CAD build for the part. Positions are in the model's coordinates, mm. Coordinates: 2 decimals unless noted, no trailing zeros. Order: outer loops, then holes, each group sorted by start corner. A loop starts at its lowest first (then second) coordinate and runs counter-clockwise, first axis right, second up. Notation, with made-up numbers: (76, -36) - (108, -36) arc R16 ccw to (108, -17) - close; hole circle Ø9 at (81.5, 85.5). An arc over 180 degrees is marked (long way). Return JSON: item names as keys, results as strings.
Autodesk Inventor part; units mm, degrees
ref_plane "YZ Plane" through (0, 0, 0) normal (1, 0, 0) x (0, 1, 0)
ref_plane "XZ Plane" through (0, 0, 0) normal (0, 1, 0) x (-1, 0, 0)
ref_plane "XY Plane" through (0, 0, 0) normal (0, 0, 1) x (1, 0, 0)
sketch "Sketch1" plane through (0, 0, 0) normal (0, 1, 0) x (-1, 0, 0)
  line L0 (6.35, -3.6662) -> (0, -7.3323)
  line L1 (0, -7.3323) -> (-6.35, -3.6662)
  line L2 (-6.35, -3.6662) -> (-6.35, 3.6662)
  line L3 (-6.35, 3.6662) -> (0, 7.3323)
  line L4 (0, 7.3323) -> (6.35, 3.6662)
  line L5 (6.35, 3.6662) -> (6.35, -3.6662)
  point P0 (0, 0)
  point P1 (0, 0)
  point P2 (0, 0)
  dimension "d0" = 12.7
extrude "Extrusion1" add sketch "Sketch1" along normal blind 673.1
hole "Hole1" at (0, 0, 0) direction (0, 1, 0) diameter 4.9784 depth 25.4
sketch "Sketch2" plane through (0, 673.1, 0) normal (0, 1, 0) x (1, 0, 0)
  point P0 (0, 0)
  point P1 (0, 0)
hole "Hole2" at (0, 673.1, 0) direction (0, -1, 0) diameter 4.9784 depth 25.4
properties part number "Intake Roller Hex Shaft"
Item 1: Mould opens along Y. For faces 1 (the flat face through (0, 673.1, -3)), 2 (the flat face through (0, 0, -3)) say: released by +Y, released by -Y, zero draft, split by the parting line, or undercut.
Findings below:
{"face 1": "released by +Y", "face 2": "released by -Y"}
Item 2: Wall check: L1, parallel to X at y = 16, z = 0; L2, parallel to Z at x = 0, y = 666.5; L3, parallel to Z at x = 1.75, y = 75. Give the ranges that are in metal, low to high. Write a range as [from, to].
Findings below:
{"L1": "x = [-6.35, -2.49], [2.49, 6.35]", "L2": "z = [-7.33, -2.49], [2.49, 7.33]", "L3": "z = [-6.32, 6.32]"}
Item 3: Band-saw the part on B-B, the plane y = 81.5. List the corners of the cut face in (x, z), then the cut area to 3 significant figures.
Findings below:
{"outline": "(-6.35, -3.67) - (0, -7.33) - (6.35, -3.67) - (6.35, 3.67) - (0, 7.33) - (-6.35, 3.67) - close", "area": "140 mm²"}
Item 4: Band-saw the part on A-A, the plane z = 0. List the corners of the cut face in (x, y), then the cut area to 3 significant figures.
Findings below:
{"outline": "(-6.35, 0) - (-2.49, 0) - (-2.49, 25.4) - (2.49, 25.4) - (2.49, 0) - (6.35, 0) - (6.35, 673.1) - (2.49, 673.1) - (2.49, 647.7) - (-2.49, 647.7) - (-2.49, 673.1) - (-6.35, 673.1) - close", "area": "8,300 mm²"}
Item 5: Drop flat-ended pins along their axis: P1, Ø2.5, axis at x = 0, z = -0.5, coming from the -Y side; P2, Ø4, axis at x = 1, y = 445.5, coming from the -Z side; P3, Ø2.5, axis at x = 0, z = -0.5, coming from the +Y side. Give the stop position or say it passes through.
Findings below:
{"P1": "stops at y = 25.4", "P2": "stops at z = -7.33", "P3": "stops at y = 647.7"}
